```python
from build123d import *

# Parameters (mm, degrees)
SKETCH_1_W          = 30
SKETCH_1_H          = 100
SKETCH_1_R          = 2.75
EXTRUDE_2_DEPTH     = 8
EXTRUDE_4_DEPTH     = 16.3
CUT_EXTRUDE_1_DEPTH = 8.3
SKETCH_5_R          = 5.5
EXTRUDE_5_DEPTH     = 8.3
SKETCH_6_R          = 5.5
CUT_EXTRUDE_2_DEPTH = 7.5
SKETCH_7_R          = 4.2
SKETCH_7_R_2        = 2.2
CUT_EXTRUDE_3_DEPTH = 21.3


with BuildPart() as part:
    # 草图1 → 凸台-拉伸2 (new body)
    with BuildSketch(Plane.XY):
        with Locations((-15, 0)):
            Rectangle(SKETCH_1_W, SKETCH_1_H)
        with Locations((-15, -40)):
            Circle(SKETCH_1_R, mode=Mode.SUBTRACT)
        with Locations((-15, 40)):
            Circle(SKETCH_1_R, mode=Mode.SUBTRACT)
    extrude(amount=EXTRUDE_2_DEPTH)

    # 草图3 → 凸台-拉伸4 (add, symmetric)
    with BuildSketch(Plane(origin=(0, 0, 0), x_dir=(1, 0, 0), z_dir=(0, 1, 0))):
        Polygon((-30, 0), (58, 0), (58, -44), (52, -49), (40, -49), (-30, -16), align=None)
    extrude(amount=EXTRUDE_4_DEPTH, both=True)

    # 草图4 → 切除-拉伸1 (cut, symmetric)
    with BuildSketch(Plane(origin=(0, 0, 0), x_dir=(1, 0, 0), z_dir=(0, 1, 0))):
        Polygon((-30, -8), (0, -8), (0, 0), (58, 0), (58, -44), (52, -49), (40, -49), (-30, -16), align=None)
    extrude(amount=CUT_EXTRUDE_1_DEPTH, both=True, mode=Mode.SUBTRACT)

    # 草图5 → 凸台-拉伸5 (add, symmetric)
    with BuildSketch(Plane(origin=(0, 0, 0), x_dir=(1, 0, 0), z_dir=(0, 1, 0))):
        with Locations(Location((30, -19, 0), (0, 0, 270))):
            Circle(SKETCH_5_R)
    extrude(amount=EXTRUDE_5_DEPTH, both=True)

    # 草图6 → 切除-拉伸2 (cut, symmetric)
    with BuildSketch(Plane(origin=(0, 0, 0), x_dir=(1, 0, 0), z_dir=(0, 1, 0))):
        with Locations(Location((30, -19, 0), (0, 0, 270))):
            Circle(SKETCH_6_R)
    extrude(amount=CUT_EXTRUDE_2_DEPTH, both=True, mode=Mode.SUBTRACT)

    # 草图7 → 切除-拉伸3 (cut, symmetric)
    with BuildSketch(Plane(origin=(0, 0, 0), x_dir=(1, 0, 0), z_dir=(0, 1, 0))):
        with Locations(Location((30, -19, 0), (0, 0, 270))):
            Circle(SKETCH_7_R)
        with Locations(Location((50.364675298, -39.364675298, 0), (0, 0, 90))):
            Circle(SKETCH_7_R_2)
    extrude(amount=CUT_EXTRUDE_3_DEPTH, both=True, mode=Mode.SUBTRACT)


solid = part.part
```
Design review of the part built by this model. Coordinates are the model's own, in mm. A direction names the side the tool comes from. Give positions to 0.01 mm unless a question says otherwise; leave off trailing zeros. Order: outer loops, then holes, each group sorted by start corner. A loop starts at its lowest first (then second) coordinate and runs counter-clockwise, first axis right, second up. Notation, with made-up numbers: (39, 2) - (98, 2) arc R19 cw to (98, 21) - close; hole circle Ø5 at (-39, -20). An arc over 180 degrees is marked (long way). Use a Markdown table: item, result. Add a question column.
(1) Add section D-D on x = 30. Give the boundary of the cut face in (y, z).
(2) Add section A-A on y = -40. Give the boundary of the cut face in (x, z), then the cut area to 3 significant figures.
(3) Clearance check with flat-ended pins moving along their axes: P1, Ø3, axis at x = -2.5, y = 15, coming from the +Z side; P2, Ø2, axis at x = 30, y = 13, coming from the -Z side; P3, Ø10, axis at x = 36, z = 11.5, coming from the +Y side; P4, Ø12, axis at x = 0, z = 22.5, coming from the -Y side. State where each tip first meets the part, or that it passes through.
(4) Mouldability with a two-part tool opening along Z and no side actions: class faces 1 (the face through (-6, 1, 0)), 2 (the face through (0, 33, 4)), 3 (the face through (30.185, -11.838, 14.804)), 4 (the face through (-15, -33, 8)) as +Z half, -Z half, draft (parallel to the pull), parting line (faces both ways), or undercut.
(5) Machinability: for faces 5 (the face through (28, 7.5, 15)), 6 (the face through (35.453, -7.894, 18.284)), 7 (the face through (0, -33, 4)), 8 (the face through (-15, 33, 8)), 9 (the face through (0, 0, 4)), which of the approach directions +Z, -Z, +X, -X, +Y, -Y give a long, thin tool a straight path to every point of the face, cutting with its end or side? Answer none if there is none.
(6) Wall thickness on probe 1 along Y at (x, z) = (-15, 5.75); probe 2 along Y at (x, z) = (41, 20.5); probe 3 along Z at (x, y) = (-3, -26): over which ranges is each line inside the solid? List them lowest first. Write a range as [from, to].
(7) Add section C-C on z = 29. Give the boundary of the cut face in (x, y), then the cut area to 3 significant figures.
(8) Add section B-B on x = -13.5. Give the boundary of the cut face in (y, z), then the cut area to 3 significant figures.
Report:
| question | item | result |
|---|---|---|
| 1 | outline | (-16.3, 0) - (-8.3, 0) - (-8.3, 13.5) - (-7.5, 13.5) - (-7.5, 14.8) - (-16.3, 14.8) - close; (-16.3, 23.2) - (-7.5, 23.2) - (-7.5, 24.5) - (-8.3, 24.5) - (-8.3, 44.29) - (-16.3, 44.29) - close; (7.5, 13.5) - (8.3, 13.5) - (8.3, 0) - (16.3, 0) - (16.3, 14.8) - (7.5, 14.8) - close; (7.5, 23.2) - (16.3, 23.2) - (16.3, 44.29) - (8.3, 44.29) - (8.3, 24.5) - (7.5, 24.5) - close |
| 2 | outline | (-30, 0) - (-17.75, 0) - (-17.75, 8) - (-30, 8) - close; (-12.25, 0) - (0, 0) - (0, 8) - (-12.25, 8) - close |
| 2 | area | 196 mm² |
| 3 | P1 | stops at z = 29.67 |
| 3 | P2 | stops at z = 0 |
| 3 | P3 | stops at y = 16.3 |
| 3 | P4 | stops at y = -16.3 |
| 4 | face 1 | -Z half |
| 4 | face 2 | draft |
| 4 | face 3 | undercut |
| 4 | face 4 | +Z half |
| 5 | face 5 | +Z, -Z, +X, -X |
| 5 | face 6 | none |
| 5 | face 7 | +Z, -Z, +X, -Y |
| 5 | face 8 | +Z, +X, -X, +Y |
| 5 | face 9 | +Z, -Z, +X |
| 6 | probe 1 | y = [-50, -42.75], [-37.25, 37.25], [42.75, 50] |
| 6 | probe 2 | y = [-16.3, -8.3], [8.3, 16.3] |
| 6 | probe 3 | z = [0, 8] |
| 7 | outline | (-2.42, -16.3) - (58, -16.3) - (58, -8.3) - (-2.42, -8.3) - close; (-2.42, 8.3) - (58, 8.3) - (58, 16.3) - (-2.42, 16.3) - close |
| 7 | area | 967 mm² |
| 8 | outline | (-50, 0) - (-42.3, 0) - (-42.3, 8) - (-50, 8) - close; (-37.7, 0) - (37.7, 0) - (37.7, 8) - (16.3, 8) - (16.3, 23.78) - (8.3, 23.78) - (8.3, 8) - (-8.3, 8) - (-8.3, 23.78) - (-16.3, 23.78) - (-16.3, 8) - (-37.7, 8) - close; (42.3, 0) - (50, 0) - (50, 8) - (42.3, 8) - close |
| 8 | area | 979 mm² |
